Can you work these out from the model? Positions are in its coordinate system, mm. Face numbers are marked on the shaded views. A direction names the side the tool comes from. Round coordinates to 2 decimals unless told otherwise and drop trailing zeros. Loops run counter-clockwise (first coordinate to the right, second up) from the corner with the lowest first, then second, coordinate; pieces in that order, holes last. Notation, with made-up numbers: (27, 60.25) -> (75, 60.25) arc R30 ccw to (75, 84.25) -> close; hole circle Ø6 at (-5.5, 29.25). An arc over 180 degrees is marked (long way). Use a Markdown table: item, result.
from build123d import *

# Parameters (mm, degrees)
SKETCH1_W           = 20
SKETCH1_H           = 8.1
BOSS_EXTRUDE1_DEPTH = 3
SKETCH2_W           = 20
SKETCH2_H           = 3
BOSS_EXTRUDE2_DEPTH = 10
SKETCH3_W           = 10.2
SKETCH3_H           = 3.2
CUT_EXTRUDE1_DEPTH  = 26.191466809
FILLET1_R           = 0.4


with BuildPart() as part:
    # Sketch1 → Boss-Extrude1 (new body)
    with BuildSketch(Plane(origin=(0, 0, 0), x_dir=(1, 0, 0), z_dir=(0, 1, 0))):
        with Locations((10, -4.05)):
            Rectangle(SKETCH1_W, SKETCH1_H)
    extrude(amount=BOSS_EXTRUDE1_DEPTH)

    # Sketch2 → Boss-Extrude2 (add)
    with BuildSketch(Plane(origin=(0, 3, 0), x_dir=(1, 0, 0), z_dir=(0, 1, 0))):
        with Locations((10, -1.5)):
            Rectangle(SKETCH2_W, SKETCH2_H)
        with Locations((10, -6.6)):
            Rectangle(SKETCH2_W, SKETCH2_H)
    extrude(amount=BOSS_EXTRUDE2_DEPTH)

    # Sketch3 → Cut-Extrude1 (cut, through all)
    with BuildSketch(Plane(origin=(0, 0, 0), x_dir=(-1, 0, 0), z_dir=(0, 0, -1))):
        with Locations((-10, 3.6)):
            Rectangle(SKETCH3_W, SKETCH3_H)
    extrude(amount=-CUT_EXTRUDE1_DEPTH, mode=Mode.SUBTRACT)

    # Fillet1
    fillet1_edges = [part.edges().sort_by_distance(p)[0] for p in [
        (0, 3, 4.05),
        (0, 8, 3),
        (20, 8, 3),
        (0, 13, 1.5),
        (10, 13, 3),
        (20, 13, 1.5),
        (10, 13, 0),
        (20, 3, 4.05),
        (0, 8, 5.1),
        (20, 8, 5.1),
        (0, 13, 6.6),
        (10, 13, 8.1),
        (20, 13, 6.6),
        (10, 13, 5.1),
        (15.1, 3.6, 8.1),
        (10, 5.2, 8.1),
        (4.9, 3.6, 8.1),
        (10, 2, 8.1),
        (15.1, 3.6, 0),
        (10, 2, 0),
        (4.9, 3.6, 0),
        (10, 0, 0),
        (10, 5.2, 0),
        (20, 0, 4.05),
        (10, 0, 8.1),
        (0, 0, 4.05),
        (0, 6.5, 0),
        (20, 6.5, 0),
        (20, 6.5, 8.1),
        (0, 6.5, 8.1),
    ]]
    fillet(fillet1_edges, radius=FILLET1_R)


solid = part.part
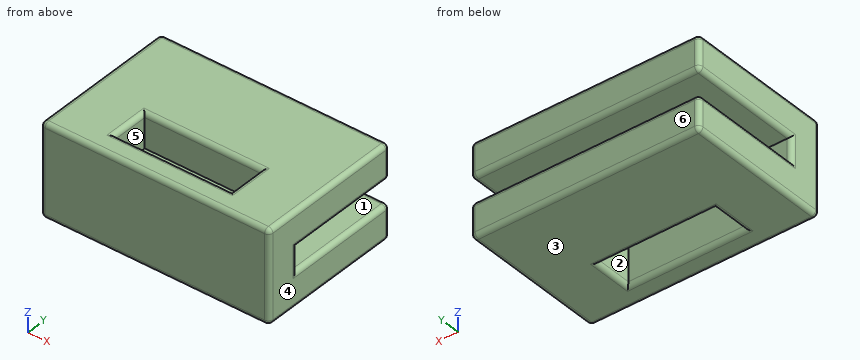
1. Which directions (+Z, -Z, +X, -X, +Y, -Y) give clear straight access to the entire face, cutting with the end or side of a thin tool? Please do the marked faces 1, 2 and 3.
Answer sheet:
| item | result |
|---|---|
| face 1 | +X, -X, +Y |
| face 2 | +Z, -Z |
| face 3 | -Z, +X, -X, +Y, -Y |
2. I need wall thicknesses on line 1 (Z direction, x = 3, y = 4.25); line 2 (Y direction, x = 9.5, z = 7.5); line 3 (X direction, y = 3, z = 0.5). Which ranges of each line are inside material? Lowest first, please.
Answer sheet:
| item | result |
|---|---|
| line 1 | z = 0 to 3, 5.1 to 8.1 |
| line 2 | y = 0 to 2, 5.2 to 13 |
| line 3 | x = 0 to 4.9, 15.1 to 20 |
3. I want a section at D-D (y = 4). Please give me the cut outline in (x, z), plus the area to 3 significant figures.
Answer sheet:
| item | result |
|---|---|
| outline | (0, 0.4) arc R0.4 ccw to (0.4, 0) -> (4.5, 0) arc R0.4 ccw to (4.9, 0.4) -> (4.9, 3) -> (0.4, 3) arc R0.4 ccw to (0, 2.6) -> close; (0, 5.5) arc R0.4 ccw to (0.4, 5.1) -> (4.9, 5.1) -> (4.9, 7.7) arc R0.4 ccw to (4.5, 8.1) -> (0.4, 8.1) arc R0.4 ccw to (0, 7.7) -> close; (15.1, 0.4) arc R0.4 ccw to (15.5, 0) -> (19.6, 0) arc R0.4 ccw to (20, 0.4) -> (20, 2.6) arc R0.4 ccw to (19.6, 3) -> (15.1, 3) -> close; (15.1, 5.1) -> (19.6, 5.1) arc R0.4 ccw to (20, 5.5) -> (20, 7.7) arc R0.4 ccw to (19.6, 8.1) -> (15.5, 8.1) arc R0.4 ccw to (15.1, 7.7) -> close |
| area | 58.4 mm² |
4. I want a section at A-A (y = 11.25). Please give me the cut outline in (x, z), plus the area to 3 significant figures.
Answer sheet:
| item | result |
|---|---|
| outline | (0, 0.4) arc R0.4 ccw to (0.4, 0) -> (19.6, 0) arc R0.4 ccw to (20, 0.4) -> (20, 2.6) arc R0.4 ccw to (19.6, 3) -> (0.4, 3) arc R0.4 ccw to (0, 2.6) -> close; (0, 5.5) arc R0.4 ccw to (0.4, 5.1) -> (19.6, 5.1) arc R0.4 ccw to (20, 5.5) -> (20, 7.7) arc R0.4 ccw to (19.6, 8.1) -> (0.4, 8.1) arc R0.4 ccw to (0, 7.7) -> close |
| area | 120 mm² |
5. If we mould it in two halves opening along X, with no side actions, what happens to the marked faces 4, 5 and 6? For each: +X half, -X half, draft (parallel to the pull), parting line (faces both ways), or undercut.
Answer sheet:
| item | result |
|---|---|
| face 4 | +X half |
| face 5 | undercut |
| face 6 | draft |
6. I want a section at C-C (z = 6). Please give me the cut outline in (x, y).
Answer sheet:
| item | result |
|---|---|
| outline | (0, 0.4) arc R0.4 ccw to (0.4, 0) -> (19.6, 0) arc R0.4 ccw to (20, 0.4) -> (20, 12.6) arc R0.4 ccw to (19.6, 13) -> (0.4, 13) arc R0.4 ccw to (0, 12.6) -> close; hole (4.9, 2) -> (15.1, 2) -> (15.1, 5.2) -> (4.9, 5.2) -> close |
7. I want a section at B-B (x = 11.75). Please give me the cut outline in (y, z), plus the area to 3 significant figures.
Answer sheet:
| item | result |
|---|---|
| outline | (0, 0.4) arc R0.4 ccw to (0.4, 0) -> (1.6, 0) arc R0.4 ccw to (2, 0.4) -> (2, 7.7) arc R0.4 ccw to (1.6, 8.1) -> (0.4, 8.1) arc R0.4 ccw to (0, 7.7) -> close; (5.2, 0.4) arc R0.4 ccw to (5.6, 0) -> (12.6, 0) arc R0.4 ccw to (13, 0.4) -> (13, 2.6) arc R0.4 ccw to (12.6, 3) -> (5.2, 3) -> close; (5.2, 5.1) -> (12.6, 5.1) arc R0.4 ccw to (13, 5.5) -> (13, 7.7) arc R0.4 ccw to (12.6, 8.1) -> (5.6, 8.1) arc R0.4 ccw to (5.2, 7.7) -> close |
| area | 62.7 mm² |
8. Will this pin go through, and if not, where does the flat tip stop? pin 1 Ø1.7 at (x, z) = (1.5, 3.5) entering from +Y.
Answer sheet:
| item | result |
|---|---|
| pin 1 | stops at y = 13 |
